The listing builds one solid part. Answer for the finished solid, in the listing's coordinates (mm). A direction names the side the tool comes from. Round coordinates to 2 decimals unless told otherwise and drop trailing zeros. Order: outer loops, then holes, each group sorted by start corner. A loop starts at its lowest first (then second) coordinate and runs counter-clockwise, first axis right, second up. Notation, with made-up numbers: (42.5, 65.5) -> (57.5, 65.5) arc R12 cw to (57.5, 69.5) -> close; hole circle Ø4 at (-20, 56). An arc over 180 degrees is marked (long way). Return JSON: item names as keys, results as strings. Group by question number.
(1) The part is cut by section D-D (y = 21). Determine the outline of the cut face in (x, z).
(2) Which of the six approach directions +Z, -Z, +X, -X, +Y, -Y give full straight-line access (tool end or side, diameter ignored) to faces 4 (the face through (31, 21, -2)), 5 (the face through (0, 0, -15))?
(3) Determine the mould class of faces 1 (the face through (0, 16, -10.25)), 2 (the face through (-23.254, 7.505, -14.687)), 3 (the face through (31.27, 19.37, 1.53)) for opening direction Y: +Y half, -Y half, draft (parallel to the pull), parting line (faces both ways), or undercut.
(4) The part is cut by section C-C (z = 15.5). Determine the outline of the cut face in (x, y).
(5) The part is cut by section B-B (x = 3). Determine the outline of the cut face in (y, z), plus the area to 3 significant figures.
(6) Each of these flat-tipped pins is pushed along its axis until it touches: pin 1 (15 mm diameter, centred on x = -9.5, y = 16, fed in from +Z); pin 2 (2 mm diameter, centred on x = 25.5, z = -2.5, fed in from -Y). Where does it stop, or does it pass through?
(7) Consider line 1 (X direction, y = 14, z = -7); line 2 (Y direction, x = -16, z = 18.5); line 3 (Z direction, x = 20, y = 33.5). Determine where each line is inside the solid, lowest interval first. Write a range as [from, to].
(8) The part is cut by section A-A (y = 10). Determine the outline of the cut face in (x, z), plus the area to 3 significant figures.
from build123d import *

# Parameters (mm, degrees)
F1_DEPTH = 35
F2_R     = 4.1
F3_DEPTH = 31
F4_DEPTH = 40.001
F5_R     = 4.1
F6_DEPTH = 19.2509998957


# Not quite as in the source:
# - ends of sketch curves that miss each other by under 0.0002 mm in the source are joined


with BuildPart() as f1:
    # F0 (on Right) → F1 (new body, symmetric)
    with BuildSketch(Plane.YZ):
        with BuildLine():
            ThreePointArc((0.6654529791, -10.3075948367), (0.1831243905, -10.6731600274), (3e-10, -11.2499998957))
            Line((3e-10, -11.2499998957), (0, -19.2499998957))
            Line((0, -19.2499998957), (40, -19.2499998957))
            Line((40, -19.2499998957), (40, 20.7500001043))
            Line((40, 20.7500001043), (32, 20.7500001043))
            ThreePointArc((32, 20.7500001043), (31.4231601317, 20.5668757138), (31.057594941, 20.0845471252))
            ThreePointArc((31.057594941, 20.0845471252), (19.2938390593, 1.456161045), (0.6654529791, -10.3075948367))
        make_face()
    extrude(amount=F1_DEPTH, both=True)

    # F2 (on Front) → F3 (cut)
    with BuildSketch(Plane.XZ):
        Polygon((-15.9000523031, -10.2499328405), (15.8999476969, -10.2499328405), (19.9999476969, -10.2499328405), (24.0999476969, -10.2499328405), (30.9999476969, -10.2499328405), (30.9999476969, 19.9232501595), (-31.0000523031, 19.9232501595), (-31.0000523031, -10.2499328405), (-24.1000523031, -10.2499328405), (-20.0000523031, -10.2499328405), align=None)
        with Locations((-20.0000523031, 0.7500671595)):
            Circle(F2_R, mode=Mode.SUBTRACT)
        with Locations((19.9999476969, 0.7500671595)):
            Circle(F2_R, mode=Mode.SUBTRACT)
        with Locations((-20.0000523031, 0.7500671595)):
            Circle(F2_R)
        with Locations((19.9999476969, 0.7500671595)):
            Circle(F2_R)
    extrude(amount=-F3_DEPTH, mode=Mode.SUBTRACT)

    # F2 (on Front) → F4 (cut, through all)
    with BuildSketch(Plane.XZ):
        with Locations((19.9999476969, 0.7500671595)):
            Circle(F2_R)
        with Locations((-20.0000523031, 0.7500671595)):
            Circle(F2_R)
    extrude(amount=-F4_DEPTH, mode=Mode.SUBTRACT)

    # F5 (on Top) → F6 (cut, through all)
    with BuildSketch(Plane.XY):
        with Locations((-20.000027626, 10)):
            Circle(F5_R)
        with Locations((19.999972374, 10)):
            Circle(F5_R)
    extrude(amount=-F6_DEPTH, mode=Mode.SUBTRACT)


solid = f1.part
Answer below:
{
 "1": {"outline": "(-35, -19.25) -> (35, -19.25) -> (35, 3.25) -> (31, 3.25) -> (31, -10.25) -> (-31, -10.25) -> (-31, 3.25) -> (-35, 3.25) -> close"},
 "2": {"face 4": "+Z, -Y", "face 5": "+Z, -Z, +X, -X, -Y"},
 "3": {"face 1": "draft", "face 2": "undercut", "face 3": "-Y half"},
 "4": {"outline": "(-35, 29.17) -> (-31, 29.17) -> (-31, 31) -> (31, 31) -> (31, 29.17) -> (35, 29.17) -> (35, 40) -> (-35, 40) -> close"},
 "5": {"outline": "(0, -19.25) -> (40, -19.25) -> (40, 20.75) -> (32, 20.75) arc R1 ccw to (31.06, 20.08) arc R50 cw to (31, 19.92) -> (31, -10.25) -> (0.83, -10.25) arc R50 cw to (0.67, -10.31) arc R1 ccw to (0, -11.25) -> close", "area": "639 mm²"},
 "6": {"pin 1": "stops at z = -10.25", "pin 2": "stops at y = 31"},
 "7": {"line 1": "x = [-35, -31], [31, 35]", "line 2": "y = [31, 40]", "line 3": "z = [-19.25, -3.35], [4.85, 20.75]"},
 "8": {"outline": "(-35, -19.25) -> (-24.1, -19.25) -> (-24.1, -10.25) -> (-31, -10.25) -> (-31, -5.86) -> (-35, -5.86) -> close; (-15.9, -19.25) -> (15.9, -19.25) -> (15.9, -10.25) -> (-15.9, -10.25) -> close; (24.1, -19.25) -> (35, -19.25) -> (35, -5.86) -> (31, -5.86) -> (31, -10.25) -> (24.1, -10.25) -> close", "area": "518 mm²"}
}
